```python
from build123d import *

# Parameters (mm, degrees)
SKETCH_W        = 90
SKETCH_H        = 30
PAD_DEPTH       = 60
SKETCH001_R     = 5
SKETCH001_R_2   = 1.5
SKETCH001_R_3   = 10.4
POCKET_DEPTH    = 60
SKETCH002_R     = 3.4
POCKET001_DEPTH = 30
SKETCH003_W     = 23
SKETCH003_H     = 23
POCKET002_DEPTH = 20
SKETCH004_W     = 15
SKETCH004_H     = 15
POCKET003_DEPTH = 5


with BuildPart() as part:
    # Sketch → Pad (new body)
    with BuildSketch(Plane.XY):
        with Locations((45, 15)):
            Rectangle(SKETCH_W, SKETCH_H)
    extrude(amount=PAD_DEPTH)

    # Sketch001 (on Face6 of Pad) → Pocket (cut)
    with BuildSketch(Plane.XY.offset(60)):
        with Locations((45, 15)):
            Circle(SKETCH001_R)
        with Locations((45, 22.5)):
            Circle(SKETCH001_R_2)
        with Locations((37.5, 15)):
            Circle(SKETCH001_R_2)
        with Locations((45, 7.5)):
            Circle(SKETCH001_R_2)
        with Locations((52.5, 15)):
            Circle(SKETCH001_R_2)
        with Locations((20.5, 15)):
            Circle(SKETCH001_R_3)
        with Locations((69.5, 15)):
            Circle(SKETCH001_R_3)
    extrude(amount=-POCKET_DEPTH, mode=Mode.SUBTRACT)

    # Sketch002 (on Face6 of Pocket) → Pocket001 (cut)
    with BuildSketch(Plane.XZ):
        with Locations((5, 53)):
            Circle(SKETCH002_R)
        with Locations((5, 7)):
            Circle(SKETCH002_R)
        with Locations((85, 53)):
            Circle(SKETCH002_R)
        with Locations((85, 7)):
            Circle(SKETCH002_R)
    extrude(amount=-POCKET001_DEPTH, mode=Mode.SUBTRACT)

    # Sketch003 (on Face4 of Pocket001) → Pocket002 (cut)
    with BuildSketch(Plane.XY.offset(60)):
        with Locations((45, 15)):
            Rectangle(SKETCH003_W, SKETCH003_H)
    extrude(amount=-POCKET002_DEPTH, mode=Mode.SUBTRACT)

    # Sketch004 (on Face10 of Pocket002) → Pocket003 (cut)
    with BuildSketch(Plane.XZ):
        with Locations((7.5, 52.5)):
            Rectangle(SKETCH004_W, SKETCH004_H)
        with Locations((82.5, 52.5)):
            Rectangle(SKETCH004_W, SKETCH004_H)
        with Locations((82.5, 7.5)):
            Rectangle(SKETCH004_W, SKETCH004_H)
        with Locations((7.5, 7.5)):
            Rectangle(SKETCH004_W, SKETCH004_H)
    extrude(amount=-POCKET003_DEPTH, mode=Mode.SUBTRACT)


solid = part.part
```
Read the model definition and answer for the solid it produces. Units are mm, in the model's axes. A direction names the side the tool comes from. Give positions to 0.01 mm unless a question says otherwise; leave off trailing zeros. Loops run counter-clockwise (first coordinate to the right, second up) from the corner with the lowest first, then second, coordinate; pieces in that order, holes last.
Item 1: For faces 1 (the flat face through (15, 2, 52)), 2 (the flat face through (82, 2, 45)), 3 (the flat face through (7, 2, 15)), determine the directions among +Z, -Z, +X, -X, +Y, -Y from which every point of the face is accessible in a straight line to the end or side of a thin tool.
Item 2: The part is cut by section C-C (x = 45). Write down the section's boundary in (y, z).
Item 3: Find the intervals of material crossed by line 1 along Z through (x, y) = (5, 13.25); line 2 along X through (y, z) = (25.5, 42.5); line 3 along Y through (x, z) = (69, 13), in increasing order.
Item 4: The part is cut by section D-D (x = 85). Write down the section's boundary in (y, z), and give its area (3 significant figures).
Item 5: The part is cut by section A-A (z = 46). Write down the section's boundary in (x, y), and give its area (3 significant figures).
Item 6: The part is cut by section B-B (y = 17.75). Write down the section's boundary in (x, z), and give its area (3 significant figures).
Item 7: Each of these flat-tipped pins is pushed along its axis until it touches: pin 1 Ø4 at (x, y) = (4.5, 3.5) entering from +Z; pin 2 Ø11 at (x, z) = (5, 7) entering from -Y; pin 3 Ø5.5 at (x, z) = (85, 7) entering from -Y; pin 4 Ø2.5 at (y, z) = (1.5, 50.5) entering from +X. Where does it stop, or does it pass through?
Item 8: The mould has two halves that part along Y. Classify faces 4 (the flat face through (44, 25, 0)), 5 (the flat face through (9, 5, 53)), 6 (the cylindrical face through (36.3, 14.1, 20.3)): released by +Y, released by -Y, zero draft, split by the parting line, or undercut.
Taken from the geometry:
1. face 1: +Z, -X, -Y
1. face 2: +Z, +X, -Y
1. face 3: -Z, -X, -Y
2. outline: (0, 0) - (6, 0) - (6, 40) - (3.5, 40) - (3.5, 60) - (0, 60) - close; (9, 0) - (10, 0) - (10, 40) - (9, 40) - close; (20, 0) - (21, 0) - (21, 40) - (20, 40) - close; (24, 0) - (30, 0) - (30, 60) - (26.5, 60) - (26.5, 40) - (24, 40) - close
3. line 1: z = 0 to 3.6, 10.4 to 49.6, 56.4 to 60
3. line 2: x = 0 to 33.5, 56.5 to 90
3. line 3: y = 0 to 4.61, 25.39 to 30
4. outline: (0, 15) - (5, 15) - (5, 10.4) - (30, 10.4) - (30, 49.6) - (5, 49.6) - (5, 45) - (0, 45) - close; (5, 0) - (30, 0) - (30, 3.6) - (5, 3.6) - close; (5, 56.4) - (30, 56.4) - (30, 60) - (5, 60) - close
4. area: 1,310 mm2
5. outline: (0, 5) - (15, 5) - (15, 0) - (75, 0) - (75, 5) - (90, 5) - (90, 30) - (0, 30) - close; hole circle Ø20.8 at (20.5, 15); hole (33.5, 3.5) - (56.5, 3.5) - (56.5, 26.5) - (33.5, 26.5) - close; hole circle Ø20.8 at (69.5, 15)
5. area: 1,340 mm2
6. outline: (0, 0) - (10.47, 0) - (10.47, 60) - (0, 60) - close; (30.53, 0) - (40.82, 0) - (40.82, 40) - (33.5, 40) - (33.5, 60) - (30.53, 60) - close; (49.18, 0) - (59.47, 0) - (59.47, 60) - (56.5, 60) - (56.5, 40) - (49.18, 40) - close; (79.53, 0) - (90, 0) - (90, 60) - (79.53, 60) - close; hole circle Ø6.8 at (5, 7); hole circle Ø6.8 at (5, 53); hole circle Ø6.8 at (85, 7); hole circle Ø6.8 at (85, 53)
6. area: 2,050 mm2
7. pin 1: stops at z = 60
7. pin 2: stops at y = 5
7. pin 3: passes through
7. pin 4: stops at x = 75
8. face 4: zero draft
8. face 5: released by -Y
8. face 6: undercut
